from build123d import *

# Parameters (mm, degrees)
SKETCH1_W           = 183
SKETCH1_H           = 183
SKETCH1_R           = 1.5
BOSS_EXTRUDE1_DEPTH = 1.6
CUT_EXTRUDE1_DEPTH  = 2
FILLET1_R           = 2
SKETCH3_R           = 1.5
CUT_EXTRUDE2_DEPTH  = 259.806027751
BOSS_EXTRUDE2_DEPTH = 1.6
SKETCH8_R           = 4
CUT_EXTRUDE4_DEPTH  = 259.806027751
BOSS_EXTRUDE4_DEPTH = 1.6
SKETCH7_R           = 1.5
CUT_EXTRUDE3_DEPTH  = 1.6


with BuildPart() as part:
    # Sketch1 → Boss-Extrude1 (new body)
    with BuildSketch(Plane(origin=(0, 0, 0), x_dir=(1, 0, 0), z_dir=(0, 1, 0))):
        with Locations((91.5, 91.5)):
            Rectangle(SKETCH1_W, SKETCH1_H)
        with Locations(Location((85.843145751, 97.156854249, 0), (0, 0, 270))):
            Circle(SKETCH1_R, mode=Mode.SUBTRACT)
        with Locations(Location((97.156854249, 97.156854249, 0), (0, 0, 270))):
            Circle(SKETCH1_R, mode=Mode.SUBTRACT)
        with Locations(Location((97.156854249, 85.843145751, 0), (0, 0, 270))):
            Circle(SKETCH1_R, mode=Mode.SUBTRACT)
        with Locations(Location((85.843145751, 85.843145751, 0), (0, 0, 270))):
            Circle(SKETCH1_R, mode=Mode.SUBTRACT)
    extrude(amount=BOSS_EXTRUDE1_DEPTH)

    # Sketch2 → Cut-Extrude1 (cut)
    with BuildSketch(Plane(origin=(0, 1.6, 0), x_dir=(1, 0, 0), z_dir=(0, 1, 0))):
        with BuildLine():
            ThreePointArc((18, 175), (15.619547443, 174.712540637), (13.375951562, 173.866689125))
            Line((13.375951562, 173.866689125), (91.5, 95.742640687))
            Line((91.5, 95.742640687), (169.624048438, 173.866689125))
            ThreePointArc((169.624048438, 173.866689125), (167.380452557, 174.712540637), (165, 175))
            Line((165, 175), (18, 175))
        make_face()
        with BuildLine():
            Line((87.257359313, 91.5), (9.133310875, 169.624048438))
            ThreePointArc((9.133310875, 169.624048438), (8.287459244, 167.38045207), (8, 164.999998998))
            Line((8, 164.999998998), (8, 18))
            ThreePointArc((8, 18), (8.287459363, 15.619547443), (9.133310875, 13.375951562))
            Line((9.133310875, 13.375951562), (87.257359313, 91.5))
        make_face()
        with BuildLine():
            Line((169.624048438, 9.133310875), (91.5, 87.257359313))
            Line((91.5, 87.257359313), (13.375951562, 9.133310875))
            ThreePointArc((13.375951562, 9.133310875), (15.619547443, 8.287459363), (18, 8))
            Line((18, 8), (165, 8))
            ThreePointArc((165, 8), (167.380452557, 8.287459363), (169.624048438, 9.133310875))
        make_face()
        with BuildLine():
            Line((173.866689125, 169.624048438), (95.742640687, 91.5))
            Line((95.742640687, 91.5), (173.866689125, 13.375951562))
            ThreePointArc((173.866689125, 13.375951562), (174.712540518, 15.619546957), (175, 17.999998998))
            Line((175, 17.999998998), (175, 165))
            ThreePointArc((175, 165), (174.712540637, 167.380452557), (173.866689125, 169.624048438))
        make_face()
    extrude(amount=-CUT_EXTRUDE1_DEPTH, mode=Mode.SUBTRACT)

    # Fillet1
    fillet1_edges = [part.edges().sort_by_distance(p)[0] for p in [
        (0, 0.8, -183),
        (183, 0.8, -183),
        (183, 0.8, 0),
        (0, 0.8, 0),
    ]]
    fillet(fillet1_edges, radius=FILLET1_R)

    # Sketch3 → Cut-Extrude2 (cut, through all)
    with BuildSketch(Plane(origin=(0, 1.6, 0), x_dir=(1, 0, 0), z_dir=(0, 1, 0))):
        with Locations(Location((4, 179, 0), (0, 0, 270))):
            Circle(SKETCH3_R)
        with Locations(Location((179, 179, 0), (0, 0, 270))):
            Circle(SKETCH3_R)
        with Locations(Location((179, 4, 0), (0, 0, 270))):
            Circle(SKETCH3_R)
        with Locations(Location((4, 4, 0), (0, 0, 270))):
            Circle(SKETCH3_R)
    extrude(amount=-CUT_EXTRUDE2_DEPTH, mode=Mode.SUBTRACT)


with BuildPart() as boss_extrude2_tool:
    # Sketch4 → Boss-Extrude2 (new body)
    with BuildSketch(Plane(origin=(0, 1.6, 0), x_dir=(1, 0, 0), z_dir=(0, 1, 0))):
        Polygon((93.5, 89.5), (175.000001002, 89.500020414), (175, 93.500020414), (93.5, 93.5), (93.5, 175), (89.5, 175), (89.5, 93.499998998), (8, 93.499978584), (8.000001002, 89.499978584), (89.5, 89.499998998), (89.5, 8), (93.5, 8), align=None)
    extrude(amount=-BOSS_EXTRUDE2_DEPTH)


with BuildPart() as part_1:
    add(part.part)


with BuildPart() as part_2:
    # Boss-Extrude2: joined with boss_extrude2_tool
    add(part_1.part.fuse(boss_extrude2_tool.part, tol=0.00001))

    # Sketch8 → Cut-Extrude4 (cut, through all)
    with BuildSketch(Plane(origin=(0, 1.6, 0), x_dir=(1, 0, 0), z_dir=(0, 1, 0))):
        with Locations(Location((91.5, 91.5, 0), (0, 0, 270))):
            Circle(SKETCH8_R)
    extrude(amount=-CUT_EXTRUDE4_DEPTH, mode=Mode.SUBTRACT)


with BuildPart() as boss_extrude4_tool:
    # Sketch6 → Boss-Extrude4 (new body)
    with BuildSketch(Plane(origin=(0, 1.6, 0), x_dir=(1, 0, 0), z_dir=(0, 1, 0))):
        Polygon((10.828426788, 89.499979292), (89.5, 10.828426753), (89.5, 8), (86.671572504, 8), (8, 86.671551831), (8, 89.499978584), align=None)
        Polygon((8, 93.500021416), (10.828426788, 93.500020708), (89.5, 172.171573247), (89.5, 175), (86.671572504, 175), (8, 96.328448169), align=None)
        Polygon((172.171573212, 93.500020708), (93.5, 172.171573247), (93.5, 175), (96.328427496, 175), (175, 96.328448169), (175, 93.500021416), align=None)
        Polygon((175, 89.499978584), (172.171573212, 89.499979292), (93.5, 10.828426753), (93.5, 8), (96.328427496, 8), (175, 86.671551831), align=None)
    extrude(amount=-BOSS_EXTRUDE4_DEPTH)


with BuildPart() as part_3:
    add(part_2.part)


with BuildPart() as part_4:
    # Boss-Extrude4: joined with boss_extrude4_tool
    add(part_3.part.fuse(boss_extrude4_tool.part, tol=0.00001))

    # Sketch7 → Cut-Extrude3 (cut)
    with BuildSketch(Plane(origin=(0, 1.6, 0), x_dir=(1, 0, 0), z_dir=(0, 1, 0))):
        with Locations(Location((29, 179, 0), (0, 0, 270))):
            Circle(SKETCH7_R)
        with Locations(Location((4, 29, 0), (0, 0, 270))):
            Circle(SKETCH7_R)
        with Locations(Location((4, 54, 0), (0, 0, 270))):
            Circle(SKETCH7_R)
        with Locations(Location((4, 79, 0), (0, 0, 270))):
            Circle(SKETCH7_R)
        with Locations(Location((4, 104, 0), (0, 0, 270))):
            Circle(SKETCH7_R)
        with Locations(Location((4, 129, 0), (0, 0, 270))):
            Circle(SKETCH7_R)
        with Locations(Location((4, 154, 0), (0, 0, 270))):
            Circle(SKETCH7_R)
        with Locations(Location((54, 179, 0), (0, 0, 270))):
            Circle(SKETCH7_R)
        with Locations(Location((79, 179, 0), (0, 0, 270))):
            Circle(SKETCH7_R)
        with Locations(Location((104, 179, 0), (0, 0, 270))):
            Circle(SKETCH7_R)
        with Locations(Location((129, 179, 0), (0, 0, 270))):
            Circle(SKETCH7_R)
        with Locations(Location((154, 179, 0), (0, 0, 270))):
            Circle(SKETCH7_R)
        with Locations(Location((179, 154, 0), (0, 0, 270))):
            Circle(SKETCH7_R)
        with Locations(Location((179, 129, 0), (0, 0, 270))):
            Circle(SKETCH7_R)
        with Locations(Location((179, 104, 0), (0, 0, 270))):
            Circle(SKETCH7_R)
        with Locations(Location((179, 79, 0), (0, 0, 270))):
            Circle(SKETCH7_R)
        with Locations(Location((179, 54, 0), (0, 0, 270))):
            Circle(SKETCH7_R)
        with Locations(Location((179, 29, 0), (0, 0, 270))):
            Circle(SKETCH7_R)
        with Locations(Location((154, 4, 0), (0, 0, 270))):
            Circle(SKETCH7_R)
        with Locations(Location((129, 4, 0), (0, 0, 270))):
            Circle(SKETCH7_R)
        with Locations(Location((104, 4, 0), (0, 0, 270))):
            Circle(SKETCH7_R)
        with Locations(Location((79, 4, 0), (0, 0, 270))):
            Circle(SKETCH7_R)
        with Locations(Location((54, 4, 0), (0, 0, 270))):
            Circle(SKETCH7_R)
        with Locations(Location((29, 4, 0), (0, 0, 270))):
            Circle(SKETCH7_R)
    extrude(amount=-CUT_EXTRUDE3_DEPTH, mode=Mode.SUBTRACT)


solid = part_4.part
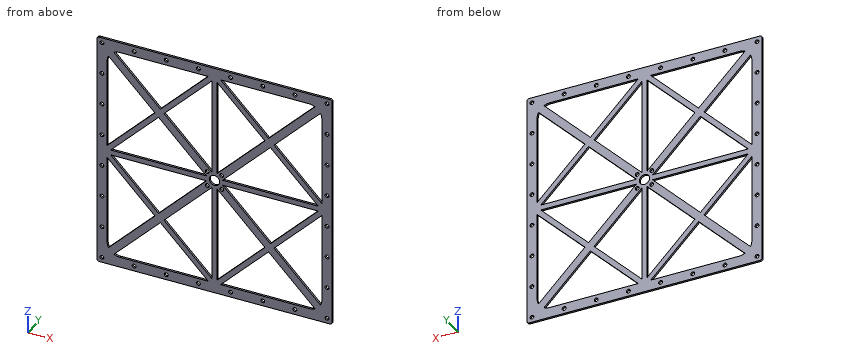
The model under review builds one solid part; all positions refer to its coordinate system, in mm. Round coordinates to 2 decimals unless told otherwise and drop trailing zeros. Write each loop counter-clockwise with the first axis right and the second up, starting at its lowest first coordinate (ties: lowest second). Pieces come first, ordered by that corner, then holes. Notation, with made-up numbers: M 84.25,-9.5 L 105.25,-9.5 A19 cw 105.25,21.5 Z; hole C 67,45.5 d3. An arc over 180 degrees is marked long. Answer as CSV lines item,"result". Start each with the question number.
Q1. Consider section C-C, the plane y = 0.55. State how many separate pieces and enclosed holes the cut face has, then the cut area to 3 significant figures.
Q2. Consider section A-A, the plane x = 20.5. Give the boundary of the cut face in (y, z).
Q3. Consider section B-B, the plane z = -74.5. Give the boundary of the cut face in (x, y), then the cut area to 3 significant figures.
Q4. Wall thickness on line 1 along Z through (x, y) = (131.5, 0.1); line 2 along Z through (x, y) = (87, 0.3); line 3 along X through (y, z) = (0.9, -47.5): over which ranges is each line inside the solid? List them lowest first.
Q5. Clearance check with a flat-ended pin moving along its axis: P1, Ø3.5, axis at x = 104, z = -4, coming from the +Y side. State where the tip first meets the part, or that it passes through.
Result set:
1,separate pieces,"1"
1,enclosed holes,"49"
1,area,"11,100 mm²"
2,outline,"M 0,-183 L 1.6,-183 L 1.6,-175 L 0,-175 Z; M 0,-166.74 L 1.6,-166.74 L 1.6,-158.26 L 0,-158.26 Z; M 0,-108.83 L 1.6,-108.83 L 1.6,-103.17 L 0,-103.17 Z; M 0,-93.5 L 1.6,-93.5 L 1.6,-89.5 L 0,-89.5 Z; M 0,-79.83 L 1.6,-79.83 L 1.6,-74.17 L 0,-74.17 Z; M 0,-24.74 L 1.6,-24.74 L 1.6,-16.26 L 0,-16.26 Z; M 0,-8 L 1.6,-8 L 1.6,0 L 0,0 Z"
3,outline,"M 0,0 L 8,0 L 8,1.6 L 0,1.6 Z; M 20.17,0 L 25.83,0 L 25.83,1.6 L 20.17,1.6 Z; M 70.26,0 L 78.74,0 L 78.74,1.6 L 70.26,1.6 Z; M 89.5,0 L 93.5,0 L 93.5,1.6 L 89.5,1.6 Z; M 104.26,0 L 112.74,0 L 112.74,1.6 L 104.26,1.6 Z; M 157.17,0 L 162.83,0 L 162.83,1.6 L 157.17,1.6 Z; M 175,0 L 183,0 L 183,1.6 L 175,1.6 Z"
3,area,"77.3 mm²"
4,line 1,"z = -183 to -175, -139.83 to -127.26, -93.5 to -89.5, -55.74 to -43.17, -8 to 0"
4,line 2,"z = -183 to -169.67, -100.24 to -98.11, -96.2 to -86.8, -84.89 to -82.76, -13.33 to 0"
4,line 3,"x = 0 to 8, 43.26 to 52.83, 89.5 to 93.5, 130.17 to 139.74, 175 to 183"
5,P1,"stops at y = 1.6"
